from build123d import *

# Parameters (mm, degrees)
CHAMFER1_SIZE = 0.5


# Read off the part's stored shape, not the designer's step: 1/4-20 Machine Threads Stud1
with BuildPart() as part:
    # Sketch1 → Revolve1 (revolve)
    with BuildSketch(Plane.XY, mode=Mode.PRIVATE) as revolve1_sk:
        Polygon((0, 0), (0, 25), (-4, 25), (-4, 15), (-6, 15), (-6, 8), (-4, 8), (-4, 0), align=None)
    revolve(revolve1_sk.sketch.rotate(Axis((0, 0, 0), (0, 1, 0)), 270), axis=Axis((0, 0, 0), (0, 1, 0)))

    # 1/4-20 Machine Threads Stud1 outline → 1/4-20 Machine Threads Stud1 (revolve, cut)
    with BuildSketch(Plane.XY):
        with BuildLine():
            Line((2.774999784, 15), (4, 15))
            Line((4, 15), (4, 25))
            Line((4, 25), (2.41935, 25))
            Line((2.41935, 25), (3.175, 24.24435))
            Line((3.175, 24.24435), (3.175, 18.592822263))
            Line((3.175, 18.592822263), (2.255384261, 17.00000108))
            ThreePointArc((2.255384261, 17.00000108), (2.195443975, 16.855292429), (2.17499946, 16.700000918))
            Line((2.17499946, 16.700000918), (2.17499946, 15.600000324))
            ThreePointArc((2.17499946, 15.600000324), (2.350735486, 15.175736026), (2.774999784, 15))
        make_face()
    revolve(axis=Axis((0, 0, 0), (0, 1, 0)), mode=Mode.SUBTRACT)

    # Chamfer1
    chamfer1_edges = [part.edges().sort_by_distance(p)[0] for p in [
        (0, 0, 4),
        (0, 8, 6),
        (0, 15, 6),
    ]]
    chamfer(chamfer1_edges, length=CHAMFER1_SIZE)


solid = part.part
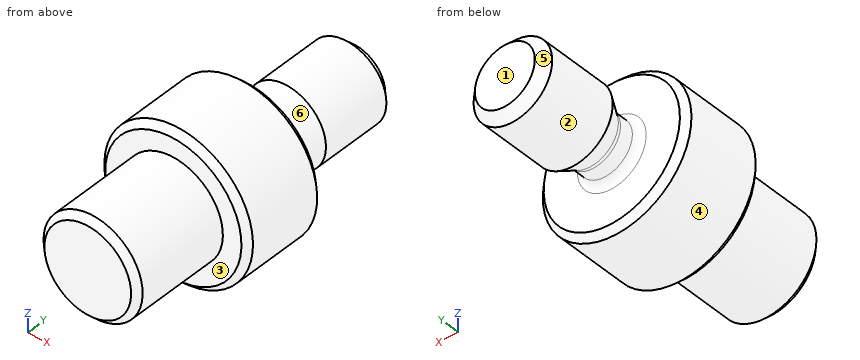
Here's how the part is built. I have some questions about the finished solid (model axes, mm). Face numbers are marked on the shaded views. A direction names the side the tool comes from. Give positions to 0.01 mm unless a question says otherwise; leave off trailing zeros. Order: outer loops, then holes, each group sorted by start corner. A loop starts at its lowest first (then second) coordinate and runs counter-clockwise, first axis right, second up. Notation, with made-up numbers: (45, 67.5) -> (56, 67.5) arc R14 ccw to (56, 88.5) -> close; hole circle Ø7 at (70, -32). An arc over 180 degrees is marked (long way). One line per item, written item: value. Start each with the question number.
1. Imagine slicing it at C-C, the plane y = 5.25. List the corners of the cut face in (x, z) for me, plus the area to 3 significant figures.
2. Imagine slicing it at D-D, the plane y = 13.5. List the corners of the cut face in (x, z) for me.
3. Imagine slicing it at B-B, the plane x = 0. List the corners of the cut face in (y, z) for me (3 decimals).
4. We'd pull the mould along Y, two halves only. Please class the marked faces 4, 5 and 6: released by +Y, released by -Y, zero draft, split by the parting line, or undercut.
5. I need wall thicknesses on probe 1 along Y at (x, z) = (4, -2); probe 2 along X at (y, z) = (23.25, 0.5); probe 3 along Y at (x, z) = (1.75, -2.75). Which ranges of each line are inside material? Lowest first, please. Write a range as from..to.
6. For the marked faces 1, 2 and 3, which set-ups out of +Z, -Z, +X, -X, +Y, -Y let a thin tool reach every point of the face, with its end or its side?
7. Imagine slicing it at A-A, the plane z = 0. List the corners of the cut face in (x, y) for me (3 decimals), plus the area to 3 significant figures.
8. Will these pins go through, and if not, where does the flat tip stop? pin 1 Ø5 at (y, z) = (15, -0.5) entering from -X; pin 2 Ø1.5 at (x, z) = (-1.5, 4) entering from +Y; pin 3 Ø1 at (y, z) = (3, 1) entering from -X; pin 4 Ø4 at (y, z) = (11.5, -3) entering from +X.
Values follow:
1. outline: circle Ø8 at (0, 0)
1. area: 50.3 mm2
2. outline: circle Ø12 at (0, 0)
3. outline: (0, -3.5) -> (0.5, -4) -> (8, -4) -> (8, -5.5) -> (8.5, -6) -> (14.5, -6) -> (15, -5.5) -> (15, -2.775) arc R0.6 cw to (15.6, -2.175) -> (16.7, -2.175) arc R0.6 cw to (17, -2.255) -> (18.593, -3.175) -> (24.244, -3.175) -> (25, -2.419) -> (25, 2.419) -> (24.244, 3.175) -> (18.593, 3.175) -> (17, 2.255) arc R0.6 cw to (16.7, 2.175) -> (15.6, 2.175) arc R0.6 cw to (15, 2.775) -> (15, 5.5) -> (14.5, 6) -> (8.5, 6) -> (8, 5.5) -> (8, 4) -> (0.5, 4) -> (0, 3.5) -> close
4. face 4: zero draft
4. face 5: released by +Y
4. face 6: undercut
5. probe 1: y = 8..15
5. probe 2: x = -3.14..3.14
5. probe 3: y = 0..15
6. face 1: +Z, -Z, +X, -X, +Y
6. face 2: +Y
6. face 3: -Y
7. outline: (-6, 8.5) -> (-5.5, 8) -> (-4, 8) -> (-4, 0.5) -> (-3.5, 0) -> (3.5, 0) -> (4, 0.5) -> (4, 8) -> (5.5, 8) -> (6, 8.5) -> (6, 14.5) -> (5.5, 15) -> (2.775, 15) arc R0.6 cw to (2.175, 15.6) -> (2.175, 16.7) arc R0.6 cw to (2.255, 17) -> (3.175, 18.593) -> (3.175, 24.244) -> (2.419, 25) -> (-2.419, 25) -> (-3.175, 24.244) -> (-3.175, 18.593) -> (-2.255, 17) arc R0.6 cw to (-2.175, 16.7) -> (-2.175, 15.6) arc R0.6 cw to (-2.775, 15) -> (-5.5, 15) -> (-6, 14.5) -> close
7. area: 205 mm2
8. pin 1: stops at x = -6
8. pin 2: stops at y = 15
8. pin 3: stops at x = -3.97
8. pin 4: stops at x = 5.92
